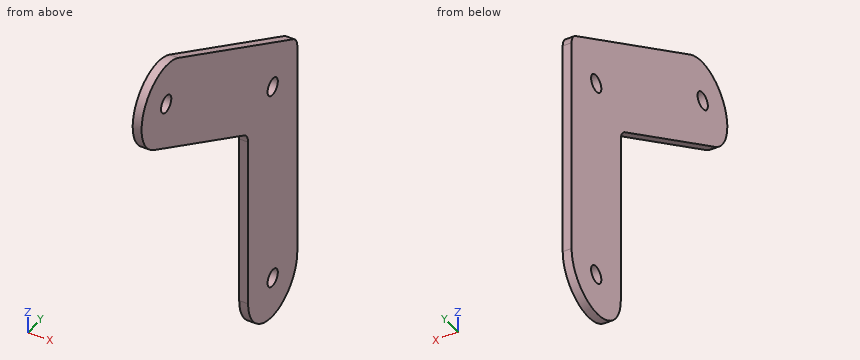
```python
from build123d import *

# Parameters (mm, degrees)
SALIENTE_EXTRUIR1_DEPTH          = 3.175
DI_METRO_DE_TALADRO_6_0_12_5_1_D = 12.5
REDONDEO1_R                      = 10


with BuildPart() as part:
    # Croquis1 → Saliente-Extruir1 (new, symmetric)
    with BuildSketch(Plane(origin=(0, 0, 0), x_dir=(0, 0, -1), z_dir=(1, 0, 0))):
        with BuildLine():
            Line((-17.320508076, 30), (150, 30))
            ThreePointArc((150, 30), (180, 0), (150, -30))
            Line((150, -30), (17.320508076, -30))
            Line((17.320508076, -30), (-49.019237886, -144.903810568))
            ThreePointArc((-49.019237886, -144.903810568), (-90, -155.884572681), (-100.980762114, -114.903810568))
            Line((-100.980762114, -114.903810568), (-17.320508076, 30))
        make_face()
    extrude(amount=SALIENTE_EXTRUIR1_DEPTH, both=True)

    # Diámetro de taladro Ø6.0 (12.5)1 (through all)
    with Locations(Plane(origin=(3.175, 0, 0), x_dir=(0, 0, -1), z_dir=(1, 0, 0))):
        with Locations((0, 0), (-75, -129.903810568), (150, 0)):
            Hole(DI_METRO_DE_TALADRO_6_0_12_5_1_D / 2)

    # Redondeo1
    redondeo1_edges = [part.edges().sort_by_distance(p)[0] for p in [
        (0, 30, 17.320508076),
        (0, -30, -17.320508076),
    ]]
    fillet(redondeo1_edges, radius=REDONDEO1_R)


solid = part.part
```
Can you work these out from the model? Positions are in its coordinate system, mm. Give positions to 0.01 mm unless a question says otherwise; leave off trailing zeros. Loops run counter-clockwise (first coordinate to the right, second up) from the corner with the lowest first, then second, coordinate; pieces in that order, holes last. Notation, with made-up numbers: M 81,43.5 L 104,43.5 A21 cw 104,53.5 Z; hole C 14.25,-19.75 d4. An arc over 180 degrees is marked long. Answer in a Markdown table with one row per item.
1. Suppose I cut it at C-C on y = 0. Write out the boundary of the cut face in (x, z) (3 decimals).
Taken from the geometry:
| item | result |
|---|---|
| outline | M -3.175,-180 L 3.175,-180 L 3.175,-156.25 L -3.175,-156.25 Z; M -3.175,-143.75 L 3.175,-143.75 L 3.175,-6.25 L -3.175,-6.25 Z; M -3.175,6.25 L 3.175,6.25 L 3.175,34.641 L -3.175,34.641 Z |
2. For pin 1 Ø3 at (x, z) = (-1, -83) entering from -Y; pin 2 Ø2 at (x, z) = (-2.5, -3) entering from -Y, each with a flat end and sliding along its axis, tell me the tip position at first contact or that it passes through.
Taken from the geometry:
| item | result |
|---|---|
| pin 1 | stops at y = -30 |
| pin 2 | stops at y = -56.54 |
3. Suppose I cut it at B-B on x = 1. Write out the boundary of the cut face in (y, z).
Taken from the geometry:
| item | result |
|---|---|
| outline | M -144.9,49.02 L -35,-14.43 A10 cw -30,-23.09 L -30,-150 A30 ccw 30,-150 L 30,11.55 A10 ccw 25,20.21 L -114.9,100.98 A30 ccw Z; hole C -129.9,75 d12.5; hole C 0,-150 d12.5; hole C 0,0 d12.5 |
4. If I drill on line 1 along Y through (x, z) = (-1, -150); line 2 along Z through (x, y) = (-2.5, 2); line 3 along Y through (x, z) = (1.25, -97), over which ranges is the centre line in solid material (lowest first)?
Taken from the geometry:
| item | result |
|---|---|
| line 1 | y = -30 to -6.25, 6.25 to 30 |
| line 2 | z = -179.93 to -155.92, -144.08 to -5.92, 5.92 to 33.49 |
| line 3 | y = -30 to 30 |
5. Suppose I cut it at A-A on z = 0. Write out the boundary of the cut face in (x, y) (3 decimals).
Taken from the geometry:
| item | result |
|---|---|
| outline | M -3.175,-60 L 3.175,-60 L 3.175,-6.25 L -3.175,-6.25 Z; M -3.175,6.25 L 3.175,6.25 L 3.175,30 L -3.175,30 Z |
6. Suppose I cut it at D-D on z = -43. Write out the boundary of the cut face in (x, y) (3 decimals), plus the area to 3 significant figures.
Taken from the geometry:
| item | result |
|---|---|
| outline | M -3.175,-30 L 3.175,-30 L 3.175,30 L -3.175,30 Z |
| area | 381 mm² |
